Source: CAD feature listing. Evaluate the final solid. Frame: model axes, mm. Coordinates: 2 decimals unless noted, no trailing zeros. Order: outer loops, then holes, each group sorted by start corner. A loop starts at its lowest first (then second) coordinate and runs counter-clockwise, first axis right, second up.
```python
from build123d import *

# Parameters (mm, degrees)
SKETCH_1_W          = 124
SKETCH_1_H          = 8
EXTRUDE_1_DEPTH     = 3
SKETCH_2_W          = 8
SKETCH_2_H          = 23
EXTRUDE_2_DEPTH     = 3
SKETCH_3_R          = 2.1
CUT_EXTRUDE_1_DEPTH = 65.915329468
FILLET_1_R          = 10
FILLET_2_R          = 4


with BuildPart() as part:
    # 草圖1 → 填料-伸長1 (new body)
    with BuildSketch(Plane.XY):
        Rectangle(SKETCH_1_W, SKETCH_1_H)
    extrude(amount=EXTRUDE_1_DEPTH)

    # 草圖2 → 填料-伸長2 (add)
    with BuildSketch(Plane.XY.offset(3)):
        with Locations((-58, 7.5)):
            Rectangle(SKETCH_2_W, SKETCH_2_H)
    extrude_2 = extrude(amount=-EXTRUDE_2_DEPTH)

    # 草圖3 → 除料-伸長1 (cut, through all)
    with BuildSketch(Plane.XY.offset(3)):
        with Locations((-58, 13)):
            Circle(SKETCH_3_R)
    cut_extrude_1 = extrude(amount=-CUT_EXTRUDE_1_DEPTH, mode=Mode.SUBTRACT)

    # 鏡射1: 填料-伸長2, 除料-伸長1 across plane
    add(extrude_2.mirror(Plane(origin=(0, 0, 0), x_dir=(0, 0, 1), z_dir=(1, 0, 0))))
    add(cut_extrude_1.mirror(Plane(origin=(0, 0, 0), x_dir=(0, 0, 1), z_dir=(1, 0, 0))), mode=Mode.SUBTRACT)

    # 圓角1
    fillet_1_edges = [part.edges().sort_by_distance(p)[0] for p in [
        (62, -4, 1.5),
        (-62, -4, 1.5),
    ]]
    fillet(fillet_1_edges, radius=FILLET_1_R)

    # 圓角2
    # the kernel refuses this fillet: 4 mm, written as the material it adds along each edge
    with BuildSketch(Plane(origin=(-54, 4, 0), x_dir=(0, 1, 0), z_dir=(0, 0, 1)), Plane(origin=(54, 4, 0), x_dir=(-1, 0, 0), z_dir=(0, 0, 1))) as fillet_2_piece_1:
        with BuildLine():
            CenterArc((FILLET_2_R, -FILLET_2_R), FILLET_2_R, 90, 90)
            Line((0, -FILLET_2_R), (0, 0))
            Line((0, 0), (FILLET_2_R, 0))
        make_face()
    extrude(amount=3)
    # the kernel refuses this fillet: 4 mm, written as the material it takes off along each edge
    with BuildSketch(Plane(origin=(62, 19, 13), x_dir=(0, -1, 0), z_dir=(0, 0, -1))) as fillet_2_2_piece_1:
        with BuildLine():
            CenterArc((FILLET_2_R, FILLET_2_R), FILLET_2_R, 180, 90)
            Line((0, FILLET_2_R), (0, 0))
            Line((0, 0), (FILLET_2_R, 0))
        make_face()
    extrude(amount=23, mode=Mode.SUBTRACT)
    with BuildSketch(Plane(origin=(54, 19, 13), x_dir=(0, -1, 0), z_dir=(0, 0, -1)), Plane(origin=(-54, 19, 13), x_dir=(-1, 0, 0), z_dir=(0, 0, -1)), Plane(origin=(-62, 19, 13), x_dir=(0, -1, 0), z_dir=(0, 0, -1))) as fillet_2_2_piece_2:
        with BuildLine():
            CenterArc((FILLET_2_R, -FILLET_2_R), FILLET_2_R, 90, 90)
            Line((0, -FILLET_2_R), (0, 0))
            Line((0, 0), (FILLET_2_R, 0))
        make_face()
    extrude(amount=23, mode=Mode.SUBTRACT)


solid = part.part
```
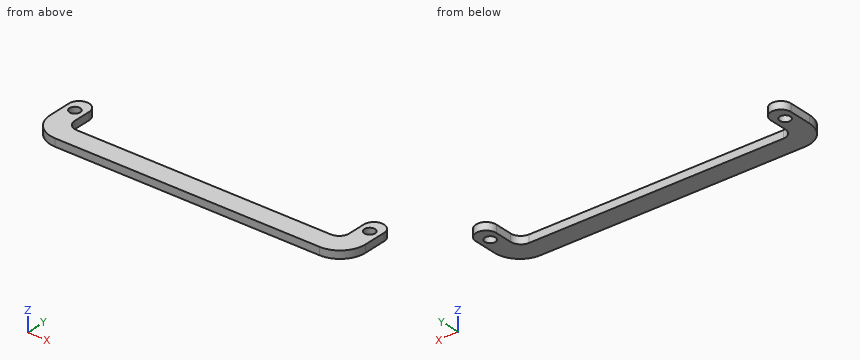
Q1. Material intervals for line 1 along X through (y, z) = (9.5, 0.8); line 2 along X through (y, z) = (13.5, 0.4); line 3 along Y through (x, z) = (-2.5, 1.45), sorted ascending.
Solutions:
line 1: x = -62 to -54, 54 to 62
line 2: x = -62 to -60.04, -55.96 to -54, 54 to 55.96, 60.04 to 62
line 3: y = -4 to 4
Q2. Pin query (flat end, axial travel): P1, Ø1, axis at y = 5, z = 1.5, coming from the -X side. Return the tip coordinate at first contact, or that it passes through.
Solutions:
P1: stops at x = -61.99
Q3. Section query B-B on x = 58. Output: boundary loops of the cut face in (y, z).
Solutions:
outline: (-2, 0) - (10.9, 0) - (10.9, 3) - (-2, 3) - close; (15.1, 0) - (19, 0) - (19, 3) - (15.1, 3) - close
Q4. Section query C-C on z = 2.3. Output: boundary loops of the cut face in (x, y).
Solutions:
outline: (-62, 6) arc R10 ccw to (-52, -4) - (52, -4) arc R10 ccw to (62, 6) - (62, 15) arc R4 ccw to (54, 15) - (54, 8) arc R4 cw to (50, 4) - (-50, 4) arc R4 cw to (-54, 8) - (-54, 15) arc R4 ccw to (-62, 15) - close; hole circle Ø4.2 at (-58, 13); hole circle Ø4.2 at (58, 13)
Q5. Section query A-A on y = 13. Output: boundary loops of the cut face in (x, z), plus the area to 3 significant figures.
Solutions:
outline: (-62, 0) - (-60.1, 0) - (-60.1, 3) - (-62, 3) - close; (-55.9, 0) - (-54, 0) - (-54, 3) - (-55.9, 3) - close; (54, 0) - (55.9, 0) - (55.9, 3) - (54, 3) - close; (60.1, 0) - (62, 0) - (62, 3) - (60.1, 3) - close
area: 22.8 mm2
Q6. Section query D-D on x = 3.5. Output: boundary loops of the cut face in (y, z).
Solutions:
outline: (-4, 0) - (4, 0) - (4, 3) - (-4, 3) - close
